from build123d import *

# Parameters (mm, degrees)
CROQUIS1_W                   = 52
CROQUIS1_H                   = 37
SALIENTE_EXTRUIR1_DEPTH      = 2
TALADRO_DE_MARGEN_PARA_M33_D = 3.4
CROQUIS9_W                   = 2
CROQUIS9_H                   = 37
SALIENTE_EXTRUIR2_DEPTH      = 42.26
CHAFL_N1_SIZE                = 2
REDONDEO1_RADIUS             = 18.5
REDONDEO1_LENGTH             = 2
TALADRO_DE_MARGEN_PARA_M34_D = 3.4
CORTAR_EXTRUIR1_DEPTH        = 70.290674697
REDONDEO3_R                  = 2
REDONDEO4_R                  = 2


with BuildPart() as part:
    # Croquis1 → Saliente-Extruir1 (new body)
    with BuildSketch(Plane(origin=(0, 0, 0), x_dir=(1, 0, 0), z_dir=(0, 1, 0))):
        Rectangle(CROQUIS1_W, CROQUIS1_H)
    extrude(amount=SALIENTE_EXTRUIR1_DEPTH)

    # Taladro de margen para M33 (through all)
    with Locations(Plane(origin=(0, 2, 0), x_dir=(1, 0, 0), z_dir=(0, 1, 0))):
        with Locations((-22, 16), (-8, 16), (6, 16), (20, 16), (-22, -16), (-8, -16), (6, -16), (20, -16)):
            Hole(TALADRO_DE_MARGEN_PARA_M33_D / 2)

    # Croquis9 → Saliente-Extruir2 (add)
    with BuildSketch(Plane(origin=(0, 2, 0), x_dir=(1, 0, 0), z_dir=(0, 1, 0))):
        with Locations((25, 0)):
            Rectangle(CROQUIS9_W, CROQUIS9_H)
    extrude(amount=SALIENTE_EXTRUIR2_DEPTH)

    # Chaflán1
    chafl_n1_edges = [part.edges().sort_by_distance(p)[0] for p in [
        (-26, 1, 18.5),
        (-26, 1, -18.5),
    ]]
    chamfer(chafl_n1_edges, length=CHAFL_N1_SIZE)

    # Redondeo1: full round fillet: the end face becomes a half cylinder, R = half its width
    redondeo1_face = Plane((25, 44.26, 0), x_dir=(-1, 0, 0), z_dir=(0, 1, 0))  # on the end face: x along it, z out of the body
    redondeo1_slab = redondeo1_face.offset(-REDONDEO1_RADIUS / 2) * Box(REDONDEO1_LENGTH, 2 * REDONDEO1_RADIUS, REDONDEO1_RADIUS, mode=Mode.PRIVATE)  # the body's end, R deep
    redondeo1_round = Plane((25, 25.76, 0), x_dir=(0, 1, 0), z_dir=(-1, 0, 0)) * Cylinder(REDONDEO1_RADIUS, REDONDEO1_LENGTH, mode=Mode.PRIVATE)  # its axis R under the face
    add(redondeo1_slab - redondeo1_round, mode=Mode.SUBTRACT)

    # Taladro de margen para M34 (through all)
    with Locations(Plane.ZY.offset(-24)):
        with Locations((-15.5, 25.76), (-7.75, 39.183393759), (7.75, 39.183393759), (15.5, 25.76), (7.75, 12.336606241), (-7.75, 12.336606241)):
            Hole(TALADRO_DE_MARGEN_PARA_M34_D / 2)

    # Croquis15 → Cortar-Extruir1 (cut, through all)
    with BuildSketch(Plane.ZY.offset(-24)):
        with BuildLine():
            Line((-6.5, 18.76), (-6.5, 32.76))
            ThreePointArc((-6.5, 32.76), (0, 39.26), (6.5, 32.76))
            Line((6.5, 32.76), (6.5, 18.76))
            ThreePointArc((6.5, 18.76), (0, 12.26), (-6.5, 18.76))
        make_face()
    extrude(amount=-CORTAR_EXTRUIR1_DEPTH, mode=Mode.SUBTRACT)

    # Redondeo3
    redondeo3_edges = [part.edges().sort_by_distance(p)[0] for p in [
        (26, 0, 0),
    ]]
    fillet(redondeo3_edges, radius=REDONDEO3_R)

    # Redondeo4
    redondeo4_edges = [part.edges().sort_by_distance(p)[0] for p in [
        (24, 2, 0),
    ]]
    fillet(redondeo4_edges, radius=REDONDEO4_R)


solid = part.part
Verification items for the finished model (mm, model axes). A direction names the side the tool comes from. Give positions to 0.01 mm unless a question says otherwise; leave off trailing zeros. Order: outer loops, then holes, each group sorted by start corner. A loop starts at its lowest first (then second) coordinate and runs counter-clockwise, first axis right, second up. Notation, with made-up numbers: M -13,-14.5 L 7,-14.5 A21 ccw 7,-3.5 Z; hole C -33.75,72 d8. An arc over 180 degrees is marked long. Use one line per item in the form item = value. Start each with the question number.
Q1. Section check A-A (x = -22). Enter the section's corners in (y, z).
Q2. Section check C-C (y = 26.5). Enter the section's corners in (x, z).
Q3. Section check D-D (z = 0.5). Enter the section's corners in (x, y), then the cut area to 3 significant figures.
Q4. Section check B-B (z = -8). Enter the section's corners in (x, y).
Q5. Access from +Z, -Z, +X, -X, +Y, -Y to the whole of each face (thin tool, end or side, straight path). Record for faces 1 (the cylindrical face through (-6.3, 0.99, 15.93)), 2 (the flat face through (-2, 2, 0)), 3 (the cylindrical face through (24.99, 39.26, -0.14)).
Q6. Mould release check, pull along X, two halves, no side actions. Record for faces 4 (the flat face through (26, 13, 4)), 5 (the cylindrical face through (18.43, 0.99, -15.35)), 6 (the cylindrical face through (25.014, 37.524, -7.381)): +X half, -X half, draft (parallel to the pull), parting line (faces both ways), or undercut.
Q7. Go/stop test with flat-tipped pins: pin 1 Ø1 at (x, y) = (25, 26.5) entering from +Z; pin 2 Ø2 at (x, z) = (1.5, 5.5) entering from +Y; pin 3 Ø5.5 at (y, z) = (12.34, 7.75) entering from -X. Record where each tip stops, or that it passes through.
Q8. Scan lines: line 1 along Z through (x, y) = (-8, 1); line 2 along Y through (x, z) = (24.7, -7.75); line 3 along X through (y, z) = (0.45, -16). Record each from-to range of solid material in increasing order. Write a range as [from, to].
Evaluation:
q1.outline = M 0,-18.5 L 2,-18.5 L 2,-17.7 L 0,-17.7 Z; M 0,-14.3 L 2,-14.3 L 2,14.3 L 0,14.3 Z; M 0,17.7 L 2,17.7 L 2,18.5 L 0,18.5 Z
q2.outline = M 24,-18.49 L 26,-18.49 L 26,-17.03 L 24,-17.03 Z; M 24,-13.97 L 26,-13.97 L 26,-6.5 L 24,-6.5 Z; M 24,6.5 L 26,6.5 L 26,13.97 L 24,13.97 Z; M 24,17.03 L 26,17.03 L 26,18.49 L 24,18.49 Z
q3.outline = M -26,0 L 24,0 A2 ccw 26,2 L 26,12.28 L 24,12.28 L 24,4 A2 cw 22,2 L -26,2 Z; M 24,39.24 L 26,39.24 L 26,44.25 L 24,44.25 Z
q3.area = 135 mm2
q4.outline = M -26,0 L 24,0 A2 ccw 26,2 L 26,10.66 L 24,10.66 L 24,4 A2 cw 22,2 L -26,2 Z; M 24,14.02 L 26,14.02 L 26,37.5 L 24,37.5 Z; M 24,40.86 L 26,40.86 L 26,42.44 L 24,42.44 Z
q5.face_1 = +Y, -Y
q5.face_2 = +Z, -Z, -X, +Y
q5.face_3 = +X, -X
q6.face_4 = +X half
q6.face_5 = undercut
q6.face_6 = draft
q7.pin_1 = 18.5
q7.pin_2 = 2
q7.pin_3 = 24
q8.line_1 = [-18.5, -17.7], [-14.3, 14.3], [17.7, 18.5]
q8.line_2 = [0.13, 10.64], [14.04, 37.48], [40.88, 42.56]
q8.line_3 = [-26, -23.7], [-20.3, -9.7], [-6.3, 4.3], [7.7, 18.3], [21.7, 25.26]
